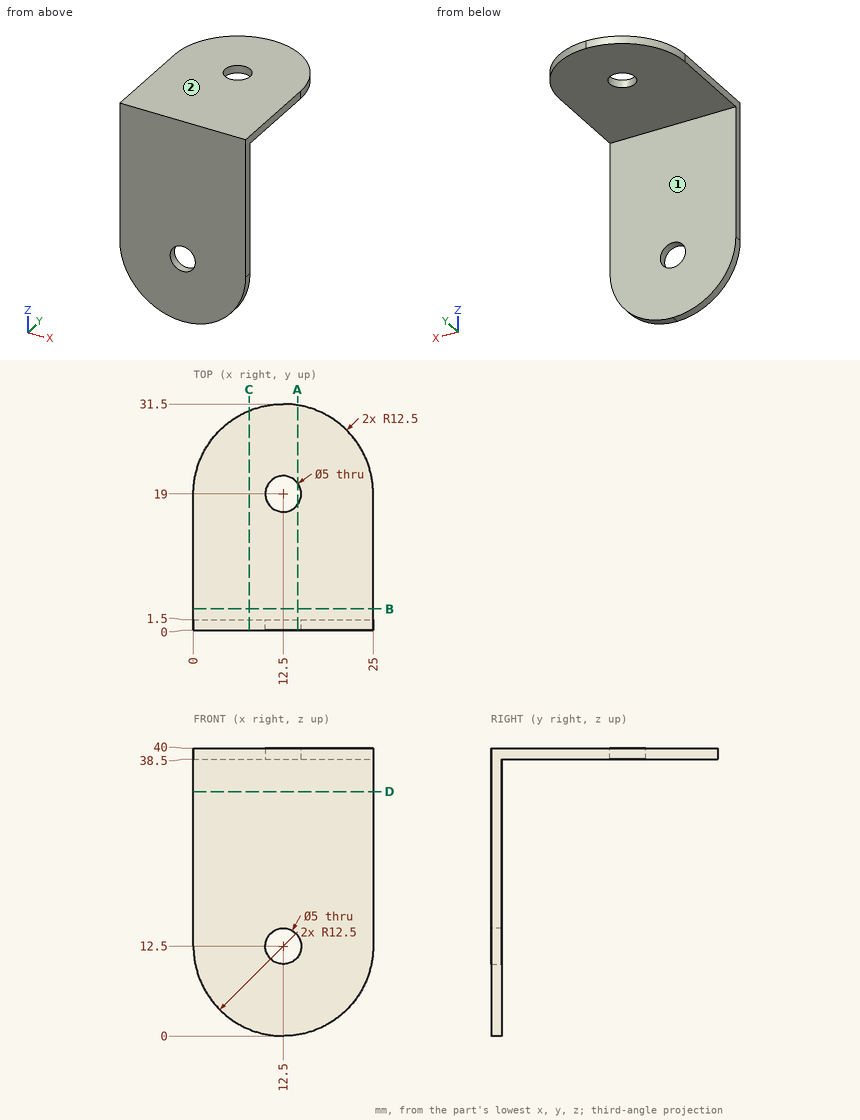
Design review of the part shown in the three views and the two pictorial views. Dimensions are in mm from the part's minimum x, y and z. A direction names the side the tool comes from. Round coordinates to 2 decimals unless told otherwise and drop trailing zeros. Write each loop counter-clockwise with the first axis right and the second up, starting at its lowest first coordinate (ties: lowest second). Pieces come first, ordered by that corner, then holes. Notation, with made-up numbers: (67.25, -27) -> (82.25, -27) arc R19 ccw to (82.25, -10) -> close; hole circle Ø5 at (76.5, 82.5). An arc over 180 degrees is marked (long way). Write item = value, one per line. Start each with the question number.
1) Take a section at A-A, the plane x = 14.5. State the section outline as (y, z) points.
2) Tool access review of the marked faces 1 and 2: name each direction out of +Z, -Z, +X, -X, +Y, -Y from which nothing blocks a thin tool from reaching the whole face with its end or side.
3) Take a section at B-B, the plane y = 3. State the section outline as (x, z) points, plus the area to 3 significant figures.
4) Clearance check with flat-ended pins moving along their axes: pin 1 (2 mm diameter, centred on x = 22, z = 23.5, fed in from +Y); pin 2 (12.5 mm diameter, centred on x = 13.5, y = 18, fed in from -Z); pin 3 (4 mm diameter, centred on y = 5, z = 8.5, fed in from +X). State where each tip first meets the part, or that it passes through.
5) Take a section at C-C, the plane x = 7.75. State the section outline as (y, z) points.
6) Wall thickness on probe 1 along X at (y, z) = (19, 39); probe 2 along Y at (x, z) = (12.5, 39.6); probe 3 along Y at (x, z) = (22, 34): over which ranges is each line inside the solid? List them lowest first. Write a range as from..to.
7) Take a section at D-D, the plane z = 34. State the section outline as (x, y) points.
Results list:
q1.outline = (0, 0.16) -> (1.5, 0.16) -> (1.5, 11) -> (0, 11) -> close; (0, 14) -> (1.5, 14) -> (1.5, 38.5) -> (17.5, 38.5) -> (17.5, 40) -> (0, 40) -> close; (20.5, 38.5) -> (31.34, 38.5) -> (31.34, 40) -> (20.5, 40) -> close
q2.face_1 = -Z, +X, -X, +Y
q2.face_2 = +Z, +X, -X, +Y, -Y
q3.outline = (0, 38.5) -> (25, 38.5) -> (25, 40) -> (0, 40) -> close
q3.area = 37.5 mm²
q4.pin_1 = 1.5
q4.pin_2 = 38.5
q4.pin_3 = through
q5.outline = (0, 0.94) -> (1.5, 0.94) -> (1.5, 38.5) -> (30.56, 38.5) -> (30.56, 40) -> (0, 40) -> close
q6.probe_1 = 0..10, 15..25
q6.probe_2 = 0..16.5, 21.5..31.5
q6.probe_3 = 0..1.5
q7.outline = (0, 0) -> (25, 0) -> (25, 1.5) -> (0, 1.5) -> close
